Design review of the part built by this model. Coordinates are the model's own, in mm. A direction names the side the tool comes from. Coordinates: 2 decimals unless noted, no trailing zeros. Write each loop counter-clockwise with the first axis right and the second up, starting at its lowest first coordinate (ties: lowest second). Pieces come first, ordered by that corner, then holes. Notation, with made-up numbers: (-39, 69) - (-16, 69) arc R19 cw to (-16, 75) - close; hole circle Ø3 at (-30, 2.5). An arc over 180 degrees is marked (long way). One line per item, written item: value.
from build123d import *

# Parameters (mm, degrees)
SKETCH2_R           = 4.7625
BOSS_EXTRUDE1_DEPTH = 158.75
BOSS_EXTRUDE2_REACH = 25.812
SKETCH1_R           = 4.7625


with BuildPart() as part:
    # Sketch2 → Boss-Extrude1 (new body, symmetric)
    with BuildSketch(Plane(origin=(0, 0, 0), x_dir=(0, 0, -1), z_dir=(1, 0, 0))):
        with Locations((-19.05, 0)):
            Circle(SKETCH2_R)
    extrude(amount=BOSS_EXTRUDE1_DEPTH, both=True)

    # Sketch1 → Boss-Extrude2 (add, up to next)
    with BuildSketch(Plane.XY, mode=Mode.PRIVATE) as boss_extrude2_sk1:
        with Locations((-127, 0)):
            Circle(SKETCH1_R)
    boss_extrude2_tool1 = extrude(boss_extrude2_sk1.sketch, amount=BOSS_EXTRUDE2_REACH, mode=Mode.PRIVATE) - part.part
    add(boss_extrude2_tool1.solids().sort_by_distance((-127, 0, 0))[0])
    # Sketch1 → Boss-Extrude2 (add, up to next)
    with BuildSketch(Plane.XY, mode=Mode.PRIVATE) as boss_extrude2_sk2:
        with Locations((127, 0)):
            Circle(SKETCH1_R)
    boss_extrude2_tool2 = extrude(boss_extrude2_sk2.sketch, amount=BOSS_EXTRUDE2_REACH, mode=Mode.PRIVATE) - part.part
    add(boss_extrude2_tool2.solids().sort_by_distance((127, 0, 0))[0])


solid = part.part
1. Consider section A-A, the plane y = 0. Write out the cut boundary in (x, z), then the cut area to 3 significant figures.
Answer block:
outline: (-158.75, 14.29) - (-131.76, 14.29) - (-131.76, 0) - (-122.24, 0) - (-122.24, 14.29) - (122.24, 14.29) - (122.24, 0) - (131.76, 0) - (131.76, 14.29) - (158.75, 14.29) - (158.75, 23.81) - (-158.75, 23.81) - close
area: 3,300 mm^2
2. Wall thickness on line 1 along X through (y, z) = (0.5, 2); line 2 along Z through (x, y) = (114, 0.75); line 3 along X through (y, z) = (3, 1.25): over which ranges is each line inside the solid? List them lowest first.
Answer block:
line 1: x = -131.74 to -122.26, 122.26 to 131.74
line 2: z = 14.35 to 23.75
line 3: x = -130.7 to -123.3, 123.3 to 130.7
3. Insertion check: pin 1 Ø2 at (x, y) = (59.5, -0.5) entering from +Z; pin 2 Ø1 at (x, y) = (-1, 3) entering from +Z; pin 3 Ø1 at (x, z) = (-16.5, 16) entering from -Y; pin 4 Ø5 at (x, y) = (43.5, -3) entering from -Z. Each pin has a flat end and moves straight along its axis. Give the tip position at first contact, or say it passes through.
Answer block:
pin 1: stops at z = 23.81
pin 2: stops at z = 23.1
pin 3: stops at y = -4.02
pin 4: stops at z = 14.31
4. Mouldability with a two-part tool opening along X and no side actions: class faces 4 (the face through (158.75, 0, 19)), 5 (the face through (131.4, -1.82, 7.27)), 6 (the face through (-158.75, 0, 19)) as released by +X, released by -X, zero draft, split by the parting line, or undercut.
Answer block:
face 4: released by +X
face 5: undercut
face 6: released by -X
5. For faces 1 (the face through (-122.6, -1.82, 7.27)), 2 (the face through (2.2, 1.4, 14.5)), 3 (the face through (-127, 0, 0)), list the 3-axis set-ups (+Z, -Z, +X, -X, +Y, -Y) from which the entire face can be reached by the end or side of a thin tool; tool diameter is ignored.
Answer block:
face 1: -Z
face 2: none
face 3: -Z, +X, -X, +Y, -Y
6. Consider section B-B, the plane z = 6.25. Write out the cut boundary in (x, y) (1 decimal).
Answer block:
outline: circle Ø9.5 at (-127, 0); circle Ø9.5 at (127, 0)
